```python
from build123d import *

# Parameters (mm, degrees)
CHAMFER_SIZE = 1


with BuildPart() as part:
    # AdditivePipe: sweep along a path in Sketch
    with BuildLine(Plane.XY) as additivepipe_path:
        Line((0, -19), (0, -12.5))
        ThreePointArc((0, -12.5), (-3.661165, -3.661165), (-12.5, 0))
        Line((-12.5, 0), (-19, 0))
    # Sketch001 → AdditivePipe (sweep)
    with BuildSketch(Plane(origin=(0, -19, 0), x_dir=(-1, 0, 0), z_dir=(0, 1, 0))):
        with BuildLine():
            Line((2.65, 2.2), (2.65, -5))
            Line((2.65, -5), (-7.35, -5))
            Line((-15, -1.8), (-7.35, -5))
            Line((-15, -1.8), (-15, 2.2))
            Line((-4.322488, 2.2), (-15, 2.2))
            Line((-4.322488, 2.2), (-4.011701, 1.661701))
            ThreePointArc((-4.011701, 1.661701), (-2.35, -2.35), (-0.688299, 1.661701))
            Line((-0.377512, 2.2), (-0.688299, 1.661701))
            Line((2.65, 2.2), (-0.377512, 2.2))
        make_face()
    sweep(path=additivepipe_path.line)

    # Chamfer
    chamfer_edges = [part.edges().sort_by_distance(p)[0] for p in [
        (-2.65, -15.75, -5),
        (-2.65, -15.75, 2.2),
        (15, -15.75, 2.2),
    ]]
    chamfer(chamfer_edges, length=CHAMFER_SIZE)


solid = part.part
```
Work out the finished part from the listing and answer in its coordinate system (mm). A direction names the side the tool comes from. Give positions to 0.01 mm unless a question says otherwise; leave off trailing zeros. Loops run counter-clockwise (first coordinate to the right, second up) from the corner with the lowest first, then second, coordinate; pieces in that order, holes last. Notation, with made-up numbers: M -35,-7.5 L -31,-7.5 A21 cw -31,18.5 Z; hole C 59,-12 d6. An arc over 180 degrees is marked long. One line per item, written item: value. Start each with the question number.
1. Find the intervals of material crossed by probe 1 along X at (y, z) = (-17.25, 0); probe 2 along Y at (x, z) = (-16, -1); probe 3 along Y at (x, z) = (-8, -1.75), in increasing order.
2. Which of the six approach directions +Z, -Z, +X, -X, +Y, -Y give full straight-line access (tool end or side, diameter ignored) to faces 1 (the face through (-15.7, -2.14, -4.51)), 2 (the face through (-3.231, -3.433, 2.047)), 3 (the face through (-15.7, -2.14, 1.71))?
3. Find section A-A (y = -13.5). Give the vertices of the cut face in (x, z).
4. Determine the mould class of faces 4 (the face through (2.43, -15.7, -2.35)), 5 (the face through (1, 1, 2.2)), 6 (the face through (-2.65, -16, -1)) for opening direction X: released by +X, released by -X, zero draft, split by the parting line, or undercut.
5. Each of these flat-tipped pins is pushed along its axis until it touches: P1, Ø4, axis at x = -17, z = 0, coming from the -Y side; P2, Ø2.5, axis at y = -14.5, z = -1.5, coming from the -X side; P3, Ø2, axis at x = -12, z = -4, coming from the -Y side. Where does it stop, or does it pass through?
6. Find section B-B (z = -3.5). Give the vertices of the cut face in (x, y).
Reported:
1. probe 1: x = -2.65 to 0, 4.7 to 15
1. probe 2: y = -2.65 to 0.22, 4.48 to 15
1. probe 3: y = -3.74 to 0, 3.29 to 14.63
2. face 1: -Z, -X, -Y
2. face 2: +Z
2. face 3: +Z, -X, -Y
3. outline: M -2.65,-4 L -1.65,-5 L 7.35,-5 L 15,-1.8 L 15,1.2 L 14,2.2 L 4.32,2.2 L 4.01,1.66 A2.35 cw long 0.69,1.66 L 0.38,2.2 L -1.65,2.2 L -2.65,1.2 Z
4. face 4: undercut
4. face 5: zero draft
4. face 6: released by -X
5. P1: stops at y = -2.65
5. P2: stops at x = -2.65
5. P3: stops at y = -2.76
6. outline: M -19,-2.65 L -12.5,-2.65 A9.85 cw -2.65,-12.5 L -2.65,-19 L 10.94,-19 L 10.94,-12.5 A23.44 ccw -12.5,10.94 L -19,10.94 Z
